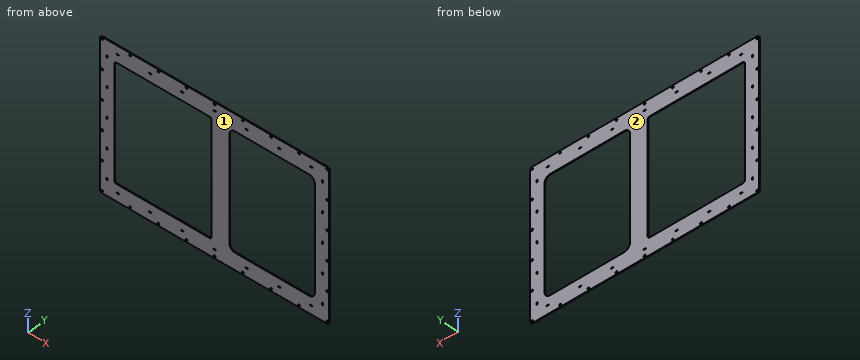
from build123d import *

# Parameters (mm, degrees)
SKETCH_1_W                  = 1165
SKETCH_1_H                  = 760
SKETCH_1_W_2                = 494
SKETCH_1_H_2                = 590
SKETCH_1_W_3                = 435
EXTRUDE_1_DEPTH             = 2
FILLET_1_R                  = 10
FILLET_2_R                  = 30
SKETCH_2_R                  = 5
CUT_EXTRUDE_1_DEPTH         = 696.501437813
PATTERN_LINEAR_1_COUNT      = 6
PATTERN_LINEAR_1_PITCH      = 148
PATTERN_LINEAR_1_COUNT_DIR2 = 9
PATTERN_LINEAR_1_PITCH_DIR2 = 143.125
SKETCH_3_W                  = 12
SKETCH_3_H                  = 4
SKETCH_3_W_2                = 4
SKETCH_3_H_2                = 12
CUT_EXTRUDE_2_DEPTH         = 696.501437813


with BuildPart() as part:
    # Эскиз1 → Бобышка-Вытянуть1 (new, symmetric)
    with BuildSketch(Plane(origin=(0, 0, 0), x_dir=(1, 0, 0), z_dir=(0, 1, 0))):
        Rectangle(SKETCH_1_W, SKETCH_1_H)
        with Locations((-262.5, 0)):
            Rectangle(SKETCH_1_W_2, SKETCH_1_H_2, mode=Mode.SUBTRACT)
        with Locations((292, 0)):
            Rectangle(SKETCH_1_W_3, SKETCH_1_H_2, mode=Mode.SUBTRACT)
    extrude(amount=EXTRUDE_1_DEPTH, both=True)

    # Скругление1
    fillet_1_edges = [part.edges().sort_by_distance(p)[0] for p in [
        (-509.5, 0, -295),
        (-509.5, 0, 295),
        (-15.5, 0, 295),
        (-15.5, 0, -295),
        (582.5, 0, 380),
        (-582.5, 0, 380),
        (-582.5, 0, -380),
        (582.5, 0, -380),
    ]]
    fillet(fillet_1_edges, radius=FILLET_1_R)

    # Скругление2
    fillet_2_edges = [part.edges().sort_by_distance(p)[0] for p in [
        (74.5, 0, -295),
        (74.5, 0, 295),
        (509.5, 0, 295),
        (509.5, 0, -295),
    ]]
    fillet(fillet_2_edges, radius=FILLET_2_R)

    # Эскиз2 → Вырез-Вытянуть1 (cut, through all)
    with BuildSketch(Plane(origin=(0, 2, 0), x_dir=(1, 0, 0), z_dir=(0, 1, 0))):
        with Locations(Location((-572.5, -370, 0), (0, 0, 270))):
            Circle(SKETCH_2_R)
    cut_extrude_1 = extrude(amount=-CUT_EXTRUDE_1_DEPTH, mode=Mode.SUBTRACT)

    # Линейный массив1: Cut-Extrude 1 6 × 9, 25 skipped
    with Locations(*[(j * PATTERN_LINEAR_1_PITCH_DIR2, 0, -i * PATTERN_LINEAR_1_PITCH) for i in range(PATTERN_LINEAR_1_COUNT) for j in range(PATTERN_LINEAR_1_COUNT_DIR2) if (i, j) not in ((0, 0), (1, 1), (1, 2), (1, 3), (1, 4), (1, 5), (1, 6), (1, 7), (2, 1), (2, 2), (2, 3), (2, 4), (2, 5), (2, 6), (2, 7), (3, 1), (3, 2), (3, 3), (3, 4), (3, 5), (3, 6), (3, 7), (4, 1), (4, 2), (4, 3), (4, 4))]):
        add(cut_extrude_1, mode=Mode.SUBTRACT)

    # Эскиз3 → Вырез-Вытянуть2 (cut, through all)
    with BuildSketch(Plane(origin=(0, 2, 0), x_dir=(1, 0, 0), z_dir=(0, 1, 0))):
        with Locations((492, 337)):
            Rectangle(SKETCH_3_W, SKETCH_3_H)
        with Locations((328, 337)):
            Rectangle(SKETCH_3_W, SKETCH_3_H)
        with Locations((0, 337)):
            Rectangle(SKETCH_3_W, SKETCH_3_H)
        with Locations((164, 337)):
            Rectangle(SKETCH_3_W, SKETCH_3_H)
        with Locations((-492, 337)):
            Rectangle(SKETCH_3_W, SKETCH_3_H)
        with Locations((-164, 337)):
            Rectangle(SKETCH_3_W, SKETCH_3_H)
        with Locations((-328, 337)):
            Rectangle(SKETCH_3_W, SKETCH_3_H)
        with Locations((492, -337)):
            Rectangle(SKETCH_3_W, SKETCH_3_H)
        with Locations((328, -337)):
            Rectangle(SKETCH_3_W, SKETCH_3_H)
        with Locations((0, -337)):
            Rectangle(SKETCH_3_W, SKETCH_3_H)
        with Locations((164, -337)):
            Rectangle(SKETCH_3_W, SKETCH_3_H)
        with Locations((-492, -337)):
            Rectangle(SKETCH_3_W, SKETCH_3_H)
        with Locations((-164, -337)):
            Rectangle(SKETCH_3_W, SKETCH_3_H)
        with Locations((-328, -337)):
            Rectangle(SKETCH_3_W, SKETCH_3_H)
        with Locations((-548, 149)):
            Rectangle(SKETCH_3_W_2, SKETCH_3_H_2)
        with Locations((-548, 298)):
            Rectangle(SKETCH_3_W_2, SKETCH_3_H_2)
        with Locations((-548, -149)):
            Rectangle(SKETCH_3_W_2, SKETCH_3_H_2)
        with Locations((-548, 0)):
            Rectangle(SKETCH_3_W_2, SKETCH_3_H_2)
        with Locations((-548, -298)):
            Rectangle(SKETCH_3_W_2, SKETCH_3_H_2)
        with Locations((548, -149)):
            Rectangle(SKETCH_3_W_2, SKETCH_3_H_2)
        with Locations((548, -298)):
            Rectangle(SKETCH_3_W_2, SKETCH_3_H_2)
        with Locations((548, 149)):
            Rectangle(SKETCH_3_W_2, SKETCH_3_H_2)
        with Locations((548, 0)):
            Rectangle(SKETCH_3_W_2, SKETCH_3_H_2)
        with Locations((548, 298)):
            Rectangle(SKETCH_3_W_2, SKETCH_3_H_2)
    extrude(amount=-CUT_EXTRUDE_2_DEPTH, mode=Mode.SUBTRACT)


solid = part.part
Read the model definition and answer for the solid it produces. Units are mm, in the model's axes. Face numbers are marked on the shaded views. Give positions to 0.01 mm unless a question says otherwise; leave off trailing zeros. Write each loop counter-clockwise with the first axis right and the second up, starting at its lowest first coordinate (ties: lowest second). Pieces come first, ordered by that corner, then holes. Notation, with made-up numbers: (-31, 62) - (-3, 62) arc R34 ccw to (-3, 100) - close; hole circle Ø2 at (-26.75, 34). An arc over 180 degrees is marked (long way). Answer in a Markdown table with one row per item. Add a question column.
Item 1: Section A-A, the plane z = 92 is taken. Write down the section's boundary in (x, y).
Item 2: A flat-ended cylindrical pin translates along its axis: P1, Ø9, axis at x = 572.5, z = 74, coming from the +Y side. Find the tip coordinate at first contact, or state that the pin passes through.
Item 3: Section C-C, the plane y = 0.25 is taken. Count the separate pieces of the cut face and the enclosed holes in it, and give its area (3 significant figures).
Item 4: Determine the mould class of the marked faces 1 and 2 for opening direction Y: pulls with the +Y half, pulls with the -Y half, needs draft (parallel to the pull), parting line crosses it, or undercut.
Item 5: Find the intervals of material crossed by L1, parallel to X at y = -0.2, z = 135.5; L2, parallel to X at y = 1.7, z = 144.5; L3, parallel to Z at x = 167, y = 0.3, in increasing order.
Item 6: Section B-B, the plane x = -231 is taken. Write down the section's boundary in (y, z), and give its area (3 significant figures).
Recorded:
| question | item | result |
|---|---|---|
| 1 | outline | (-582.5, -2) - (-509.5, -2) - (-509.5, 2) - (-582.5, 2) - close; (-15.5, -2) - (74.5, -2) - (74.5, 2) - (-15.5, 2) - close; (509.5, -2) - (582.5, -2) - (582.5, 2) - (509.5, 2) - close |
| 2 | P1 | passes through |
| 3 | separate pieces | 1 |
| 3 | enclosed holes | 52 |
| 3 | area | 335,000 mm2 |
| 4 | face 1 | pulls with the -Y half |
| 4 | face 2 | pulls with the +Y half |
| 5 | L1 | x = -582.5 to -509.5, -15.5 to 74.5, 509.5 to 582.5 |
| 5 | L2 | x = -582.5 to -550, -546 to -509.5, -15.5 to 74.5, 509.5 to 546, 550 to 582.5 |
| 5 | L3 | z = -380 to -339, -335 to -295, 295 to 335, 339 to 380 |
| 6 | outline | (-2, -380) - (2, -380) - (2, -295) - (-2, -295) - close; (-2, 295) - (2, 295) - (2, 380) - (-2, 380) - close |
| 6 | area | 680 mm2 |
